Could you check a few things on this drawing? It's one solid part, dimensions in mm from its lowest x, y, z. A direction names the side the tool comes from. Round coordinates to 2 decimals unless told otherwise and drop trailing zeros. Write each loop counter-clockwise with the first axis right and the second up, starting at its lowest first coordinate (ties: lowest second). Pieces come first, ordered by that corner, then holes. Notation, with made-up numbers: (33, 83.25) -> (79, 83.25) arc R26 cw to (79, 113.25) -> close; hole circle Ø1 at (52, -30). An arc over 180 degrees is marked (long way). Return JSON: item names as keys, results as strings.
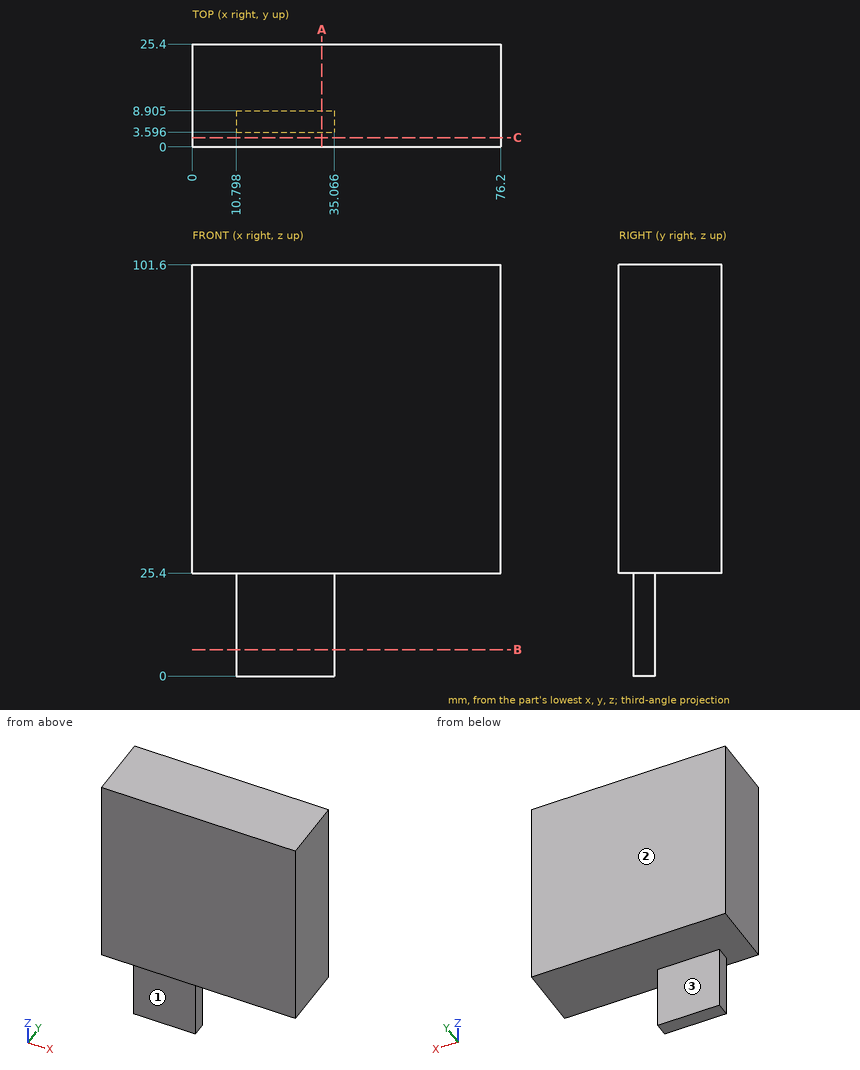
1) I want a section at C-C, the plane y = 2.25. Please give me the cut outline in (x, z), and give its area (3 significant figures).
Return value:
{"outline": "(0, 25.4) -> (76.2, 25.4) -> (76.2, 101.6) -> (0, 101.6) -> close", "area": "5,810 mm²"}
2) If I drill on probe 1 along Z at (x, y) = (31.5, 11.5); probe 2 along Y at (x, z) = (14, 4.5) (1 decimal); probe 3 along X at (y, z) = (6.75, 7), over which ranges is the centre line in solid material (lowest first)? Write a range as [from, to].
Return value:
{"probe 1": "[25.4, 101.6]", "probe 2": "[3.6, 8.9]", "probe 3": "[10.8, 35.07]"}
3) I want a section at A-A, the plane x = 32. Please give me the cut outline in (y, z) (1 decimal), and give its area (3 significant figures).
Return value:
{"outline": "(0, 25.4) -> (3.6, 25.4) -> (3.6, 0) -> (8.9, 0) -> (8.9, 25.4) -> (25.4, 25.4) -> (25.4, 101.6) -> (0, 101.6) -> close", "area": "2,070 mm²"}
4) Will these pins go through, and if not, where does the flat tip stop? pin 1 Ø4 at (y, z) = (5.5, 11.5) entering from +X; pin 2 Ø4 at (y, z) = (5, 7) entering from -X; pin 3 Ø12.5 at (x, y) = (37, 18) entering from -Z.
Return value:
{"pin 1": "x = 35.07", "pin 2": "x = 10.8", "pin 3": "z = 25.4"}
5) For the marked faces 1, 2 and 3, which set-ups out of +Z, -Z, +X, -X, +Y, -Y let a thin tool reach every point of the face, with its end or its side?
Return value:
{"face 1": "-Z, +X, -X, -Y", "face 2": "+Z, -Z, +X, -X, +Y", "face 3": "-Z, +X, -X, +Y"}
6) I want a section at B-B, the plane z = 6.5. Please give me the cut outline in (x, y) (1 decimal).
Return value:
{"outline": "(10.8, 3.6) -> (35.1, 3.6) -> (35.1, 8.9) -> (10.8, 8.9) -> close"}
